```python
from build123d import *

# Parameters (mm, degrees)
SKETCH1_W           = 20
SKETCH1_H           = 11
SKETCH1_R           = 1.6
BOSS_EXTRUDE1_DEPTH = 42
SKETCH2_W           = 20
SKETCH2_H           = 30.5
CUT_EXTRUDE1_DEPTH  = 11
FILLET1_R           = 2


with BuildPart() as part:
    # Sketch1 → Boss-Extrude1 (new body)
    with BuildSketch(Plane(origin=(0, 0, 0), x_dir=(1, 0, 0), z_dir=(0, 1, 0))):
        Rectangle(SKETCH1_W, SKETCH1_H)
        with Locations((5.25, 0)):
            Circle(SKETCH1_R, mode=Mode.SUBTRACT)
        with Locations((-5.25, 0)):
            Circle(SKETCH1_R, mode=Mode.SUBTRACT)
        Polygon((10, -5.5), (-10, -5.5), (-30, -5.5), (-30, -11.5), (10, -11.5), align=None)
    extrude(amount=BOSS_EXTRUDE1_DEPTH)

    # Sketch2 → Cut-Extrude1 (cut)
    with BuildSketch(Plane(origin=(0, 0, -5.5), x_dir=(-1, 0, 0), z_dir=(0, 0, -1))):
        with Locations((0, 21)):
            Rectangle(SKETCH2_W, SKETCH2_H)
    extrude(amount=-CUT_EXTRUDE1_DEPTH, mode=Mode.SUBTRACT)

    # Fillet1
    fillet1_edges = [part.edges().sort_by_distance(p)[0] for p in [
        (-10, 0, 11.5),
        (-20, 0, 5.5),
        (-10, 0, 0),
        (-10, 39.125, 5.5),
        (-10, 39.125, -5.5),
        (10, 39.125, -5.5),
        (-10, 42, 0),
        (-10, 2.875, 5.5),
        (-10, 2.875, -5.5),
        (10, 2.875, -5.5),
        (-20, 42, 5.5),
        (-10, 42, 11.5),
    ]]
    fillet(fillet1_edges, radius=FILLET1_R)


solid = part.part
```
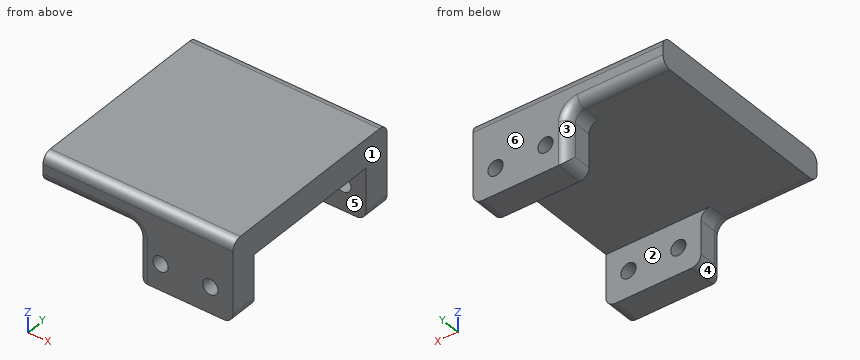
The model under review builds one solid part; all positions refer to its coordinate system, in mm. Face numbers are marked on the shaded views. A direction names the side the tool comes from. Give positions to 0.01 mm unless a question says otherwise; leave off trailing zeros. Write each loop counter-clockwise with the first axis right and the second up, starting at its lowest first coordinate (ties: lowest second). Pieces come first, ordered by that corner, then holes. Notation, with made-up numbers: (-1.75, 62) - (12.25, 62) arc R37 cw to (12.25, 99) - close; hole circle Ø1 at (-31.75, -18.75). An arc over 180 degrees is marked (long way). Answer in a Markdown table with one row per item. Add a question column.
1. We need section D-D on z = 2.5. Write out the cut boundary in (x, y).
2. Tool access review of the marked faces 1, 2 and 3: name each direction out of +Z, -Z, +X, -X, +Y, -Y from which nothing blocks a thin tool from reaching the whole face with its end or side.
3. We need section B-B on z = 0. Write out the cut boundary in (x, y), then the cut area to 3 significant figures.
4. Insertion check: P1, Ø5, axis at x = -5.25, z = 0, coming from the +Y side; P2, Ø1.1, axis at y = 38, z = -0.5, coming from the -X side; P3, Ø10, axis at x = -22.5, z = 2, coming from the -Y side. Each pin has a flat end and moves straight along its axis. Give the tip position at first contact, or say it passes through.
5. We need section A-A on x = -5.25. Write out the cut boundary in (y, z), then the cut area to 3 significant figures.
6. We need section C-C on y = 5. Write out the cut boundary in (x, z).
7. Draft analysis for pull direction Y (two halves, no side actions). For the marked faces 4, 5 and 6, state which applies: +Y half, -Y half, draft (parallel to the pull), parting line (faces both ways), or undercut.
8. Wall thickness on line 1 along X through (y, z) = (2.05, 0); line 2 along Y through (x, z) = (-6, 3.5); line 3 along Z through (x, y) = (5.25, 2.95): over which ranges is each line inside the solid? List them lowest first. Write a range as [from, to].
Ans:
| question | item | result |
|---|---|---|
| 1 | outline | (-10, 2) arc R2 ccw to (-8, 0) - (10, 0) - (10, 5.75) - (-10, 5.75) - close; (-10, 36.25) - (10, 36.25) - (10, 42) - (-8, 42) arc R2 ccw to (-10, 40) - close |
| 2 | face 1 | +Z, -Z, +X, +Y, -Y |
| 2 | face 2 | -Z, +X, -X |
| 2 | face 3 | -Z, -X, +Y |
| 3 | outline | (-10, 2) arc R2 ccw to (-8, 0) - (-6.85, 0) - (-6.85, 5.75) - (-10, 5.75) - close; (-10, 36.25) - (-6.85, 36.25) - (-6.85, 42) - (-8, 42) arc R2 ccw to (-10, 40) - close; (-3.65, 0) - (3.65, 0) - (3.65, 5.75) - (-3.65, 5.75) - close; (-3.65, 36.25) - (3.65, 36.25) - (3.65, 42) - (-3.65, 42) - close; (6.85, 0) - (10, 0) - (10, 5.75) - (6.85, 5.75) - close; (6.85, 36.25) - (10, 36.25) - (10, 42) - (6.85, 42) - close |
| 3 | area | 155 mm^2 |
| 4 | P1 | stops at y = 42 |
| 4 | P2 | stops at x = -10 |
| 4 | P3 | stops at y = 0.06 |
| 5 | outline | (0, -5.5) - (5.75, -5.5) - (5.75, -1.6) - (0, -1.6) - close; (0, 1.6) - (5.75, 1.6) - (5.75, 5.5) - (36.25, 5.5) - (36.25, 1.6) - (42, 1.6) - (42, 9.5) arc R2 ccw to (40, 11.5) - (2, 11.5) arc R2 ccw to (0, 9.5) - close; (36.25, -5.5) - (42, -5.5) - (42, -1.6) - (36.25, -1.6) - close |
| 5 | area | 340 mm^2 |
| 6 | outline | (-30, 5.5) - (-12, 5.5) arc R2 cw to (-10, 3.5) - (-10, -3.5) arc R2 ccw to (-8, -5.5) - (8, -5.5) arc R2 ccw to (10, -3.5) - (10, 11.5) - (-30, 11.5) - close; hole circle Ø3.2 at (-5.25, 0); hole circle Ø3.2 at (5.25, 0) |
| 7 | face 4 | draft |
| 7 | face 5 | undercut |
| 7 | face 6 | +Y half |
| 8 | line 1 | x = [-10, -6.85], [-3.65, 3.65], [6.85, 10] |
| 8 | line 2 | y = [0, 5.75], [36.25, 42] |
| 8 | line 3 | z = [-5.5, -1.6], [1.6, 11.5] |
